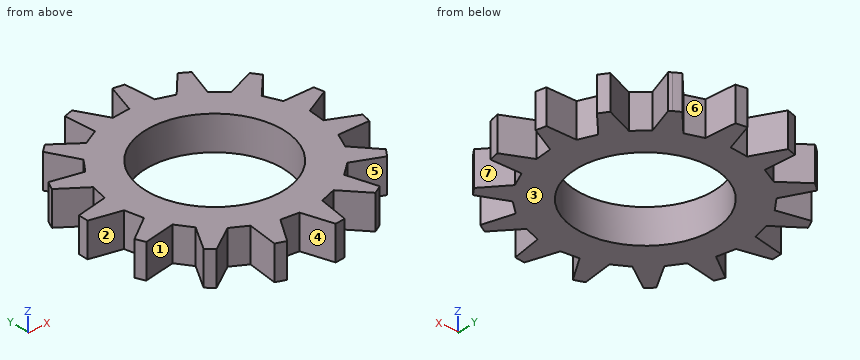
from build123d import *

# Parameters (mm, degrees)
F1_DEPTH = 2.54
F4_D     = 10.16
F4_DEPTH = 2.54
F4_TIP   = 3.0523719447


with BuildPart() as f1:
    # F0 (on Top) → F1 (new body)
    with BuildSketch(Plane.XY):
        with BuildLine():
            Line((-6.8331683087, -6.8155120711), (-6.2978819926, -7.3050655915))
            Line((-6.2978819926, -7.3050655915), (-4.316461231, -5.9911443529))
            Line((-4.316461231, -5.9911443529), (-3.1834454186, -6.6520702435))
            Line((-3.1834454186, -6.6520702435), (-3.4675601543, -8.9987342074))
            Line((-3.4675601543, -8.9987342074), (-2.7476248397, -9.2706777631))
            Line((-2.7476248397, -9.2706777631), (-1.4900637669, -7.2682696548))
            Line((-1.4900637669, -7.2682696548), (-0.1799902587, -7.4061532934))
            Line((-0.1799902587, -7.4061532934), (0.53803154, -9.6603514426))
            Line((0.53803154, -9.6603514426), (1.2835661727, -9.5852906378))
            Line((1.2835661727, -9.5852906378), (1.6418913593, -7.2682696548))
            Line((1.6418913593, -7.2682696548), (2.8590536505, -6.8429019717))
            Line((2.8590536505, -6.8429019717), (4.4267883674, -8.6114303767))
            ThreePointArc((4.4267883674, -8.6114303767), (4.7621164114, -8.430624868), (5.0900724152, -8.2367682491))
            Line((5.0900724152, -8.2367682491), (4.414810271, -5.9861610474))
            Line((4.414810271, -5.9861610474), (5.416404056, -5.1173232333))
            Line((5.416404056, -5.1173232333), (7.5402496681, -6.0743578528))
            ThreePointArc((7.5402496681, -6.0743578528), (7.7785505678, -5.7660505935), (8.0042534911, -5.4484047603))
            Line((8.0042534911, -5.4484047603), (6.4974054455, -3.7073606396))
            Line((6.4974054455, -3.7073606396), (7.0467623816, -2.5027365269))
            Line((7.0467623816, -2.5027365269), (9.3462724586, -2.5298971346))
            ThreePointArc((9.3462724586, -2.5298971346), (9.4419154496, -2.145558441), (9.5217606328, -1.757629891))
            Line((9.5217606328, -1.757629891), (7.4543519629, -0.7753081489))
            Line((7.4543519629, -0.7753081489), (7.5720577138, 0.515978468))
            Line((7.5720577138, 0.515978468), (9.4118826679, 1.4620667743))
            Line((9.4118826679, 1.4620667743), (9.5596825543, 1.5380695179))
            Line((9.5596825543, 1.5380695179), (9.416678635, 2.2537417481))
            ThreePointArc((9.416678635, 2.2537417481), (9.4137978769, 2.2657444506), (9.4109018198, 2.2777434708))
            Line((9.4109018198, 2.2777434708), (7.1536707948, 2.2777434708))
            Line((7.1536707948, 2.2777434708), (6.6120580312, 3.506264905))
            Line((6.6120580312, 3.506264905), (8.1813489345, 5.1786791747))
            ThreePointArc((8.1813489345, 5.1786791747), (7.9680827327, 5.5011676894), (7.7421121151, 5.8148850701))
            Line((7.7421121151, 5.8148850701), (5.5964540897, 4.9471179465))
            Line((5.5964540897, 4.9471179465), (4.619770739, 5.8493615309))
            Line((4.619770739, 5.8493615309), (5.3694094978, 8.0347383187))
            Line((5.3694094978, 8.0347383187), (5.1664119437, 8.1891010502))
            ThreePointArc((5.1664119437, 8.1891010502), (4.9301428504, 8.3334794568), (4.6898420519, 8.4710430237))
            Line((4.6898420519, 8.4710430237), (3.1182668573, 6.7673715214))
            Line((3.1182668573, 6.7673715214), (1.8562393493, 7.2027559673))
            Line((1.8562393493, 7.2027559673), (1.6558854627, 9.5211366727))
            Line((1.6558854627, 9.5211366727), (0.9290533371, 9.6379483438))
            ThreePointArc((0.9290533371, 9.6379483438), (0.8909600606, 9.641544407), (0.8528528712, 9.6449899099))
            Line((0.8528528712, 9.6449899099), (0.1102985869, 7.3744878367))
            Line((0.1102985869, 7.3744878367), (-1.2349347684, 7.2456887003))
            Line((-1.2349347684, 7.2456887003), (-2.4185909857, 9.3696708082))
            Line((-2.4185909857, 9.3696708082), (-3.128865287, 9.1543172047))
            Line((-3.128865287, 9.1543172047), (-2.9428471919, 6.8132407112))
            Line((-2.9428471919, 6.8132407112), (-4.1615320816, 6.1761889411))
            Line((-4.1615320816, 6.1761889411), (-6.016344287, 7.5866191285))
            ThreePointArc((-6.016344287, 7.5866191285), (-6.321753073, 7.3340729793), (-6.6165717429, 7.0692408894))
            Line((-6.6165717429, 7.0692408894), (-5.4735798935, 4.9287530222))
            Line((-5.4735798935, 4.9287530222), (-6.2615627322, 3.8819453014))
            Line((-6.2615627322, 3.8819453014), (-8.5762331436, 4.3989693402))
            Line((-8.5762331436, 4.3989693402), (-8.9240014984, 3.7051745846))
            Line((-8.9240014984, 3.7051745846), (-7.0272791194, 2.3135405903))
            Line((-7.0272791194, 2.3135405903), (-7.3407024127, 1.0249859563))
            Line((-7.3407024127, 1.0249859563), (-9.6667165043, 0.5547796031))
            ThreePointArc((-9.6667165043, 0.5547796031), (-9.6809513806, 0.1799131703), (-9.6806547422, -0.1952233199))
            Line((-9.6806547422, -0.1952233199), (-7.4054314828, -0.7064821591))
            Line((-7.4054314828, -0.7064821591), (-7.1172324763, -2.0714243811))
            Line((-7.1172324763, -2.0714243811), (-9.0316843933, -3.4364557412))
            Line((-9.0316843933, -3.4364557412), (-8.7383911794, -4.1093048652))
            Line((-8.7383911794, -4.1093048652), (-6.3862953563, -3.6664897539))
            Line((-6.3862953563, -3.6664897539), (-5.6214329554, -4.7591500254))
            Line((-5.6214329554, -4.7591500254), (-6.8331683087, -6.8155120711))
        make_face()
    extrude(amount=F1_DEPTH)


with BuildPart() as f1_1:
    # F3: moved
    add(f1.part)

    # F4
    with Locations(Plane(origin=(0, 0, 0), x_dir=(1, 0, 0), z_dir=(0, 0, -1))):
        with Locations((0, 0)):
            Hole(F4_D / 2, depth=F4_DEPTH)
            with Locations((0, 0, -(F4_DEPTH + F4_TIP / 2))):  # 118° drill point
                Cone(0, F4_D / 2, F4_TIP, mode=Mode.SUBTRACT)


solid = f1_1.part
Can you work these out from the model? Positions are in its coordinate system, mm. Face numbers are marked on the shaded views. A direction names the side the tool comes from. Give positions to 0.01 mm unless a question says otherwise; leave off trailing zeros. Loops run counter-clockwise (first coordinate to the right, second up) from the corner with the lowest first, then second, coordinate; pieces in that order, holes last. Notation, with made-up numbers: (-32, 13) -> (-2, 13) arc R26 cw to (-2, 46) -> close; hole circle Ø11 at (-24, -12.5). An arc over 180 degrees is marked (long way). Use one line per item in the form item = value.
1) Will these pins go through, and if not, where does the flat tip stop? pin 1 (1.1 mm diameter, centred on x = 8.5, z = 1, fed in from +Y); pin 2 (1.5 mm diameter, centred on x = -1, y = 7.5, fed in from +Z); pin 3 (8 mm diameter, centred on x = 0, y = 0, fed in from -Z).
Answers:
pin_1 = 5.53
pin_2 = 2.54
pin_3 = through
2) We'd pull the mould along Y, two halves only. Please class the marked faces 1, 2, 3 and 4: released by +Y, released by -Y, zero draft, split by the parting line, or undercut.
Answers:
face_1 = undercut
face_2 = undercut
face_3 = zero draft
face_4 = released by -Y
3) If we section it at A-A (y = -2.75): Please give me the cut outline in (x, z).
Answers:
outline = (-8.07, 0) -> (-4.27, 0) -> (-4.27, 2.54) -> (-8.07, 2.54) -> close; (4.27, 0) -> (6.93, 0) -> (6.93, 2.54) -> (4.27, 2.54) -> close
4) For the marked faces 5, 6 and 7, which set-ups out of +Z, -Z, +X, -X, +Y, -Y let a thin tool reach every point of the face, with its end or its side?
Answers:
face_5 = +Z, -Z, -Y
face_6 = +Z, -Z, +Y
face_7 = +Z, -Z, +X
5) I need wall thicknesses on line 1 along Y through (x, z) = (-7.5, 1.6); line 2 along X through (y, z) = (-7.75, 2.2); line 3 along Y through (x, z) = (-7.75, 0.3). Which ranges of each line are inside material? Lowest first, please.
Answers:
line_1 = -3.88 to -2.34, -0.69 to 0.99, 2.66 to 4.16
line_2 = -3.32 to -1.79, -0.07 to 1.57, 3.66 to 4.94
line_3 = -3.92 to -2.52, -0.63 to 0.94, 2.84 to 4.21
6) If we section it at B-B (x = 2.25): Please give me the cut outline in (y, z), plus the area to 3 significant figures.
Answers:
outline = (-7.06, 0) -> (-4.55, 0) -> (-4.55, 2.54) -> (-7.06, 2.54) -> close; (4.55, 0) -> (7.07, 0) -> (7.07, 2.54) -> (4.55, 2.54) -> close
area = 12.7 mm²
